Autodesk Inventor part; units mm, degrees
ref_plane "YZ Plane" through (0, 0, 0) normal (1, 0, 0) x (0, 1, 0)
ref_plane "XZ Plane" through (0, 0, 0) normal (0, 1, 0) x (-1, 0, 0)
ref_plane "XY Plane" through (0, 0, 0) normal (0, 0, 1) x (1, 0, 0)
sketch "Sketch1" plane through (0, 0, 0) normal (0, 1, 0) x (-1, 0, 0)
  line L0 (-56.25, 58.1) -> (56.25, 58.1)
  line L1 (56.25, 58.1) -> (56.25, -58.1)
  line L2 (56.25, -58.1) -> (-56.25, -58.1)
  line L3 (-56.25, -58.1) -> (-56.25, 58.1)
  line L4 (-56.25, 58.1) -> (56.25, -58.1) construction
  line L5 (56.25, 58.1) -> (-56.25, -58.1) construction
  point P0 (0, 0)
  dimension "d0" = 112.5
  dimension "d1" = 116.2
extrude "Extrusion1" add sketch "Sketch1" along normal blind 5
sketch "Sketch3" plane through (0, 5, 0) normal (0, 1, 0) x (1, 0, 0)
  line L0 (-67.6879, -53.1) -> (61.6788, -53.1) construction
  line L1 (51.25, 64.0604) -> (51.25, -69.5663) construction
  line L2 (-51.25, 74.598) -> (-51.25, -75.8441) construction
  line L3 (-56.25, 58.1) -> (-56.25, -58.1) construction
  line L4 (56.25, -58.1) -> (56.25, 58.1) construction
  line L5 (-56.25, -58.1) -> (56.25, -58.1) construction
  line L6 (-98.6283, 41.4) -> (135.891, 41.4) construction
  line L7 (-92.1264, -8.6) -> (97.1034, -8.6) construction
  line L8 (56.25, 58.1) -> (-56.25, 58.1) construction
  point P0 (0, 0)
  point P1 (51.25, 41.4)
  point P2 (51.25, -8.6)
  point P3 (-51.25, 41.4)
  point P4 (-51.25, -8.6)
  point P5 (-43.95, -53.1)
  point P6 (2.65, -53.1)
  point P7 (51.25, -53.1)
  dimension "d21" = 5
  dimension "d22" = 5
  dimension "d23" = 5
  dimension "d34" = 12.3
  dimension "d35" = 58.9
  dimension "d36" = 107.5
  dimension "d37" = 49.5
  dimension "d38" = 99.5
hole "Hole1" at (51.25, 5, -41.4) at (51.25, 5, 8.6) at (-51.25, 5, -41.4) at (-51.25, 5, 8.6) at (-43.95, 5, 53.1) at (2.65, 5, 53.1) at (51.25, 5, 53.1) direction (0, -1, 0) diameter 3.8 end through all
properties part number "Bottle Base Plate"
Build history of the part. All positions in model axes, mm. Coordinates: 2 decimals unless noted, no trailing zeros. Order: outer loops, then holes, each group sorted by start corner. A loop starts at its lowest first (then second) coordinate and runs counter-clockwise, first axis right, second up. Notation, with made-up numbers: M -24.75,78 L 0.25,78 A32 ccw 0.25,109 Z; hole C 56.25,66.5 d6. An arc over 180 degrees is marked long. One line per question, with ' | ' between items. Start each with the question number.
Q1. Saw through at B-B (z = -41.4). List the corners of the cut face in (x, y).
Q2. Saw through at A-A (x = -43.95). List the corners of the cut face in (y, z).
Q3. Two-plate mould, pull along Z, no slides. Class faces 1 (the face through (1, 2, 58.1)), 2 (the face through (53.105, 2.465, 8.188)), 3 (the face through (1, 0, 1)): +Z half, -Z half, draft (parallel to the pull), parting line (faces both ways), or undercut.
Q4. Probe L1, parallel to X at y = 3.8, z = 8.6; L2, parallel to X at y = 3.4, z = 53.1; L3, parallel to Z at x = 51.25, y = 1.6. List the from-to ranges inside material, lowest first. Write a range as from..to.
Check values:
1) outline: M -56.25,0 L -53.15,0 L -53.15,5 L -56.25,5 Z; M -49.35,0 L 49.35,0 L 49.35,5 L -49.35,5 Z; M 53.15,0 L 56.25,0 L 56.25,5 L 53.15,5 Z
2) outline: M 0,-58.1 L 5,-58.1 L 5,51.2 L 0,51.2 Z; M 0,55 L 5,55 L 5,58.1 L 0,58.1 Z
3) face 1: +Z half | face 2: undercut | face 3: draft
4) L1: x = -56.25..-53.15, -49.35..49.35, 53.15..56.25 | L2: x = -56.25..-45.85, -42.05..0.75, 4.55..49.35, 53.15..56.25 | L3: z = -58.1..-43.3, -39.5..6.7, 10.5..51.2, 55..58.1
